```python
from build123d import *

# Parameters (mm, degrees)
SKETCH1_W           = 28.575
SKETCH1_H           = 16.256
SKETCH1_R           = 2.4892
SKETCH1_R_2         = 1.75
BOSS_EXTRUDE1_DEPTH = 12.7
SKETCH2_W           = 36.398054667
SKETCH2_H           = 7.747
CUT_EXTRUDE1_DEPTH  = 3.175
SKETCH3_W           = 33.032622038
SKETCH3_H           = 11.5824
CUT_EXTRUDE2_DEPTH  = 3.175
SKETCH4_R           = 3.7465
CUT_EXTRUDE3_DEPTH  = 3.6322
FILLET1_R           = 5.08
SKETCH5_R           = 4.7625
CUT_EXTRUDE4_DEPTH  = 35.227383569


with BuildPart() as part:
    # Sketch1 → Boss-Extrude1 (new body)
    with BuildSketch(Plane(origin=(0, 0, 0), x_dir=(1, 0, 0), z_dir=(0, 1, 0))):
        with Locations((14.2875, 8.128)):
            Rectangle(SKETCH1_W, SKETCH1_H)
        with Locations(Location((23.495, 8.128, 0), (0, 0, 270))):
            Circle(SKETCH1_R, mode=Mode.SUBTRACT)
        with Locations(Location((12.4714, 8.128, 0), (0, 0, 270))):
            Circle(SKETCH1_R_2, mode=Mode.SUBTRACT)
    extrude(amount=BOSS_EXTRUDE1_DEPTH)

    # Sketch2 → Cut-Extrude1 (cut)
    with BuildSketch(Plane(origin=(0, 12.7, 0), x_dir=(1, 0, 0), z_dir=(0, 1, 0))):
        with Locations((15.783080999, 8.128)):
            Rectangle(SKETCH2_W, SKETCH2_H)
    extrude(amount=-CUT_EXTRUDE1_DEPTH, mode=Mode.SUBTRACT)

    # Sketch3 → Cut-Extrude2 (cut)
    with BuildSketch(Plane.XZ):
        with Locations((15.449592918, -8.128)):
            Rectangle(SKETCH3_W, SKETCH3_H)
    extrude(amount=-CUT_EXTRUDE2_DEPTH, mode=Mode.SUBTRACT)

    # Sketch4 → Cut-Extrude3 (cut)
    with BuildSketch(Plane.XZ.offset(-3.175)):
        with Locations(Location((12.4714, -8.128, 0), (0, 0, 270))):
            Circle(SKETCH4_R)
    extrude(amount=-CUT_EXTRUDE3_DEPTH, mode=Mode.SUBTRACT)

    # Fillet1
    fillet1_edges = [part.edges().sort_by_distance(p)[0] for p in [
        (28.575, 6.35, -16.256),
        (28.575, 6.35, 0),
    ]]
    fillet(fillet1_edges, radius=FILLET1_R)

    # Sketch5 → Cut-Extrude4 (cut, through all)
    with BuildSketch(Plane(origin=(0, 9.525, 0), x_dir=(1, 0, 0), z_dir=(0, 1, 0))):
        with Locations((23.495, 8.128)):
            Circle(SKETCH5_R)
    extrude(amount=CUT_EXTRUDE4_DEPTH, mode=Mode.SUBTRACT)


solid = part.part
```
Input: part model. Units: mm. Frame: model coordinates. A direction names the side the tool comes from. Give positions to 0.01 mm unless a question says otherwise; leave off trailing zeros. Order: outer loops, then holes, each group sorted by start corner. A loop starts at its lowest first (then second) coordinate and runs counter-clockwise, first axis right, second up.
1. Draft query along Z for faces 1 (the face through (0, 6, -8)), 2 (the face through (12, 6, -16.256)), 3 (the face through (12, 6.807, -10)), 4 (the face through (27, 11, -12.002)). Return one class per face: released by +Z, released by -Z, zero draft, split by the parting line, or undercut.
Computed:
face 1: zero draft
face 2: released by -Z
face 3: undercut
face 4: undercut
2. Line query: probe 1 along Z at (x, y) = (5.75, 12); probe 2 along X at (y, z) = (4, -10) (3 decimals); probe 3 along X at (y, z) = (5.25, -6.5) (3 decimals). Output: solid intervals per line, ascending.
Computed:
probe 1: z = -16.26 to -12, -4.25 to 0
probe 2: x = 0 to 9.226, 15.717 to 21.854, 25.136 to 28.575
probe 3: x = 0 to 9.097, 15.846 to 21.612, 25.378 to 28.575
3. Cut plane A-A (y = 11.75). Return loops of the section in (x, z) (1 decimal).
Computed:
outline: (0, -16.3) - (23.5, -16.3) arc R5.1 ccw to (28.5, -12) - (26.3, -12) arc R4.8 cw to (20.7, -12) - (0, -12) - close; (0, -4.3) - (20.7, -4.3) arc R4.8 cw to (26.3, -4.3) - (28.5, -4.3) arc R5.1 ccw to (23.5, 0) - (0, 0) - close
4. Cut plane C-C (x = 24.75). Return loops of the section in (y, z) (3 decimals), and give its area (3 significant figures).
Computed:
outline: (0, -16.099) - (12.7, -16.099) - (12.7, -12.722) - (9.525, -12.722) - (9.525, -10.278) - (3.175, -10.278) - (3.175, -13.919) - (0, -13.919) - close; (0, -2.337) - (3.175, -2.337) - (3.175, -5.978) - (9.525, -5.978) - (9.525, -3.534) - (12.7, -3.534) - (12.7, -0.157) - (0, -0.157) - close
area: 109 mm2
5. Cut plane D-D (y = 2). Return loops of the section in (x, z) (3 decimals).
Computed:
outline: (0, -16.256) - (23.495, -16.256) arc R5.08 ccw to (27.771, -13.919) - (0, -13.919) - close; (0, -2.337) - (27.771, -2.337) arc R5.08 ccw to (23.495, 0) - (0, 0) - close
6. Cut plane B-B (x = 19.5). Return loops of the section in (y, z) (1 decimal).
Computed:
outline: (0, -16.3) - (12.7, -16.3) - (12.7, -12) - (9.5, -12) - (9.5, -4.3) - (12.7, -4.3) - (12.7, 0) - (0, 0) - (0, -2.3) - (3.2, -2.3) - (3.2, -13.9) - (0, -13.9) - close
7. Set-up query: faces 5 (the face through (27, 11, -4.254)), 6 (the face through (23.454, 11.09, -3.366)), 7 (the face through (14, 2, -2.337)). Return all of +Z, -Z, +X, -X, +Y, -Y with unobstructed straight access to the full face (end or side cutting, diameter ignored); none if empty.
Computed:
face 5: +X, -X, +Y
face 6: +Y
face 7: +X, -X, -Y
8. Pin query (flat end, axial travel): pin 1 Ø8 at (x, z) = (12, -8.5) entering from -Y (3 decimals); pin 2 Ø2.5 at (x, y) = (27.5, 11) entering from +Z; pin 3 Ø4 at (x, z) = (23.495, -8.128) entering from +Y; pin 4 Ø6.5 at (x, z) = (12.47, -8.13) entering from +Y (3 decimals). Return the tip coordinate at first contact, or that it passes through.
Computed:
pin 1: stops at y = 3.175
pin 2: stops at z = -0.81
pin 3: passes through
pin 4: stops at y = 9.525
